from build123d import *

# Parameters (mm, degrees)
BOSS_EXTRUDE1_DEPTH = 4
SHELL1_START        = 1
SHELL1_DEPTH        = 3
SKETCH2_R           = 1.25
SKETCH2_R_2         = 0.75
SKETCH2_R_3         = 1
CUT_EXTRUDE1_DEPTH  = 10
SKETCH3_W           = 10.665868521
SKETCH3_H           = 3
BOSS_EXTRUDE2_DEPTH = 1
SKETCH4_R           = 0.9
BOSS_EXTRUDE3_DEPTH = 3
SKETCH5_R           = 0.75
CUT_EXTRUDE2_DEPTH  = 3


# Read off the part's stored shape, not the designer's step: Shell1
with BuildPart() as part:
    # Sketch1 → Boss-Extrude1 (new body)
    with BuildSketch(Plane.XY):
        with BuildLine():
            Line((-17.017879978, -7), (6.982120022, -7))
            Line((6.982120022, -7), (6.982120022, -5.5))
            Line((6.982120022, -5.5), (6.982120022, -4.5))
            Line((6.982120022, -4.5), (7.982120022, -4.5))
            Line((7.982120022, -4.5), (8.482120022, -4.5))
            ThreePointArc((8.482120022, -4.5), (9.189226803, -4.207106781), (9.482120022, -3.5))
            Line((9.482120022, -3.5), (9.482120022, -0.5))
            ThreePointArc((9.482120022, -0.5), (9.189226803, 0.207106781), (8.482120022, 0.5))
            Line((8.482120022, 0.5), (7.858116823, 0.5))
            ThreePointArc((7.858116823, 0.5), (7.220739384, 0.72944825), (6.87585222, 1.3125))
            ThreePointArc((6.87585222, 1.3125), (1.68605895, 6.793909421), (-5.464373249, 4.375))
            ThreePointArc((-5.464373249, 4.375), (-5.811985297, 4.098612181), (-6.244997998, 4))
            Line((-6.244997998, 4), (-14.017879978, 4))
            ThreePointArc((-14.017879978, 4), (-16.139200322, 3.121320344), (-17.017879978, 1))
            Line((-17.017879978, 1), (-17.017879978, -7))
        make_face()
    extrude(amount=BOSS_EXTRUDE1_DEPTH)

    # Shell1 outline → Shell1 (cut)
    with BuildSketch(Plane.XY.offset(SHELL1_START)):
        with BuildLine():
            Line((-16.017879978, 1), (-16.017879978, -7))
            Line((-16.017879978, -7), (5.982120022, -7))
            Line((5.982120022, -7), (5.982120022, -3.5))
            Line((5.982120022, -3.5), (8.482120022, -3.5))
            Line((8.482120022, -3.5), (8.482120022, -0.5))
            Line((8.482120022, -0.5), (7.858116823, -0.5))
            ThreePointArc((7.858116823, -0.5), (6.583361944, -0.041103501), (5.893587617, 1.125))
            ThreePointArc((5.893587617, 1.125), (1.445193386, 5.823350932), (-4.683748499, 3.75))
            ThreePointArc((-4.683748499, 3.75), (-5.378972594, 3.197224362), (-6.244997998, 3))
            Line((-6.244997998, 3), (-14.017879978, 3))
            ThreePointArc((-14.017879978, 3), (-15.43209354, 2.414213562), (-16.017879978, 1))
        make_face()
    extrude(amount=SHELL1_DEPTH, mode=Mode.SUBTRACT)

    # Sketch2 → Cut-Extrude1 (cut)
    with BuildSketch(Plane.XY.offset(1)):
        Circle(SKETCH2_R)
        with Locations((-12.017879978, -4.8)):
            Circle(SKETCH2_R_2)
        with Locations((-7.517879978, -3.5)):
            Circle(SKETCH2_R_3)
        Polygon((-5.517879978, 1), (-4.017879978, 1), (-3.017879978, -2), (-4.517879978, -2), align=None)
    extrude(amount=-CUT_EXTRUDE1_DEPTH, mode=Mode.SUBTRACT)

    # Sketch3 → Boss-Extrude2 (add)
    with BuildSketch(Plane.XZ.offset(7)):
        with Locations((0.649185762, 2.5)):
            Rectangle(SKETCH3_W, SKETCH3_H)
    extrude(amount=-BOSS_EXTRUDE2_DEPTH)

    # Sketch4 → Boss-Extrude3 (add)
    with BuildSketch(Plane.XY.offset(1)):
        with Locations((-14.517879978, 2.936491673)):
            Circle(SKETCH4_R)
        with Locations((-16.017879978, -1.5)):
            Circle(SKETCH4_R)
        with Locations((7.782120022, -0.7)):
            Circle(SKETCH4_R)
        with Locations((6.732120022, -3.7)):
            Circle(SKETCH4_R)
    extrude(amount=BOSS_EXTRUDE3_DEPTH)

    # Sketch5 → Cut-Extrude2 (cut)
    with BuildSketch(Plane.XY.offset(4)):
        with Locations((-14.517879978, 2.936491673)):
            Circle(SKETCH5_R)
        with Locations((-16.017879978, -1.5)):
            Circle(SKETCH5_R)
        with Locations((6.732120022, -3.7)):
            Circle(SKETCH5_R)
        with Locations((7.782120022, -0.7)):
            Circle(SKETCH5_R)
    extrude(amount=-CUT_EXTRUDE2_DEPTH, mode=Mode.SUBTRACT)


solid = part.part
Here's how the part is built. I have some questions about the finished solid (model axes, mm). A direction names the side the tool comes from. Give positions to 0.01 mm unless a question says otherwise; leave off trailing zeros. Order: outer loops, then holes, each group sorted by start corner. A loop starts at its lowest first (then second) coordinate and runs counter-clockwise, first axis right, second up. Notation, with made-up numbers: (2, 30) -> (43, 30) arc R21 cw to (43, 55) -> close; hole circle Ø7 at (7.5, 54). An arc over 180 degrees is marked (long way). One line per item, written item: value. Start each with the question number.
1. Imagine slicing it at B-B, the plane z = 0.4. Count the separate pieces of the cut face and the enclosed holes in it, plus the area to 3 significant figures.
2. We'd pull the mould along Y, two halves only. Please class faces 1 (the face through (9.181, -4.215, 1.972)), 2 (the face through (-15.83, 1.85, 2.48)), 3 (the face through (-10, 4, 2)), 4 (the face through (-17.018, -3, 2)): released by +Y, released by -Y, zero draft, split by the parting line, or undercut.
3. Will these pins go through, and if not, where does the flat tip stop? pin 1 Ø1.2 at (x, y) = (7.78, -0.7) entering from +Z; pin 2 Ø0.9 at (y, z) = (-5.5, 2) entering from +X; pin 3 Ø0.7 at (x, z) = (8, 2.5) entering from +Y.
4. I need wall thicknesses on probe 1 along Y at (x, z) = (0, 0.5); probe 2 along X at (y, z) = (-1, 1.4); probe 3 along Z at (x, y) = (2, -0.75). Which ranges of each line are inside material? Lowest first, please. Write a range as from..to.
5. For faces 5 (the face through (7.033, -0.667, 2.521)), 6 (the face through (-5, 4, 4)), 7 (the face through (-4.8, 1, 0.5)), which set-ups out of +Z, -Z, +X, -X, +Y, -Y let a thin tool reach every point of the face, with its end or its side?
6. Imagine slicing it at A-A, the plane x = 0. List the corners of the cut face in (y, z) for me.
7. Imagine slicing it at C-C, the plane x = -8.25. List the corners of the cut face in (y, z) for me, plus the area to 3 significant figures.
Values follow:
1. separate pieces: 1
1. enclosed holes: 4
1. area: 283 mm2
2. face 1: released by -Y
2. face 2: undercut
2. face 3: released by +Y
2. face 4: zero draft
3. pin 1: stops at z = 1
3. pin 2: stops at x = 6.98
3. pin 3: stops at y = 0.52
4. probe 1: y = -7..-1.25, 1.25..7
4. probe 2: x = -17.02..-16.58, -15.46..-15.27, 6.93..7.09, 8.47..9.48
4. probe 3: z = 0..1
5. face 5: +Z
5. face 6: +Z, +X, -X, +Y, -Y
5. face 7: +Z, -Z
6. outline: (-7, 0) -> (-1.25, 0) -> (-1.25, 1) -> (-6, 1) -> (-6, 4) -> (-7, 4) -> close; (1.25, 0) -> (7, 0) -> (7, 4) -> (6, 4) -> (6, 1) -> (1.25, 1) -> close
7. outline: (-7, 0) -> (-4.18, 0) -> (-4.18, 1) -> (-7, 1) -> close; (-2.82, 0) -> (4, 0) -> (4, 4) -> (3, 4) -> (3, 1) -> (-2.82, 1) -> close
7. area: 12.6 mm2
